Part model, mm, in its own coordinate system. A direction names the side the tool comes from. Round coordinates to 2 decimals unless told otherwise and drop trailing zeros. Write each loop counter-clockwise with the first axis right and the second up, starting at its lowest first coordinate (ties: lowest second). Pieces come first, ordered by that corner, then holes. Notation, with made-up numbers: (81.25, 9) -> (86.25, 9) arc R8 ccw to (86.25, 24) -> close; hole circle Ø10 at (37.5, -2). An arc over 180 degrees is marked (long way). Return JSON: item names as keys, results as strings. Group by question number.
(1) Saw through at D-D (x = -34). List the corners of the cut face in (y, z) (3 decimals), plus the area to 3 significant figures.
(2) Tool access for faces 5 (the cylindrical face through (53.513, -11.795, -23.021)), 6 (the cylindrical face through (-39.05, 11.79, -10.66)), 7 (the flat face through (-53, 0, -22.066)): list every direction of +Z, -Z, +X, -X, +Y, -Y with a clear straight run to the whole face (end or side of a thin tool).
(3) Saw through at A-A (y = 0). State how many separate pieces and enclosed holes the cut face has, plus the area to 3 significant figures.
(4) Drill centre lines: L1, parallel to X at y = 5, z = -6.5; L2, parallel to Y at x = -57, z = -29; L3, parallel to X at y = -2.25, z = -24.5. Where is each one in solid material? Low to high. Write a range as from..to.
(5) Saw through at C-C (z = -6). List the corners of the cut face in (x, y) (3 decimals), plus the area to 3 significant figures.
(6) Drop flat-ended pins along their axis: pin 1 Ø6 at (y, z) = (9.5, 7.5) entering from +X; pin 2 Ø5.5 at (y, z) = (-1, -2) entering from -X; pin 3 Ø7.5 at (x, y) = (-55, 0.5) entering from +Z. Give the stop position or say it passes through.
(7) Mould opens along X. For faces 1 (the flat face through (0, -12.7, 10)), 2 (the cylindrical face through (-39.05, -11.79, -10.66)), 3 (the cylindrical face through (61.59, -10.89, -28.37)), 4 (the cylindrical face through (-49.85, 11.79, -6.46)) say: +X half, -X half, draft (parallel to the pull), parting line (faces both ways), or undercut.
(8) Saw through at B-B (x = 0). List the corners of the cut face in (y, z) (3 decimals).
from build123d import *

# Parameters (mm, degrees)
F1_DEPTH = 12.7
F2_R     = 3.175
F3_DEPTH = 9.526
F4_R     = 6.35
F5_DEPTH = 50.801
F6_R     = 6.35
F7_R     = 3.17499


# Not quite as in the source:
# - a fillet or chamfer is up to 0.001 mm smaller than in the source, because OpenCascade refuses the exact size


with BuildPart() as f1:
    # F0 (on Front) → F1 (new body, symmetric)
    with BuildSketch(Plane.XZ):
        Polygon((-50.8, -22.066242151), (-63.5, -22.066242151), (-63.5, -31.591242151), (-38.1, -31.591242151), (-38.1, 6.508757849), (0, 6.508757849), (38.1, 6.508757849), (38.1, -31.591242151), (63.5, -31.591242151), (63.5, -22.066242151), (50.8, -22.066242151), (50.8, 19.208757849), (0, 19.208757849), (-50.8, 19.208757849), align=None)
    extrude(amount=F1_DEPTH, both=True)

    # F2 (on face) → F3 (cut, through all)
    with BuildSketch(Plane.XY.offset(-22.066242151)):
        with Locations((-57.15, 0)):
            Circle(F2_R)
        with Locations((57.15, 0)):
            Circle(F2_R)
    extrude(amount=-F3_DEPTH, mode=Mode.SUBTRACT)

    # F4 (on face) → F5 (cut, through all)
    with BuildSketch(Plane.XY.offset(19.208757849)):
        Circle(F4_R)
    extrude(amount=-F5_DEPTH, mode=Mode.SUBTRACT)

    # F6
    f6_edges = [f1.edges().sort_by_distance(p)[0] for p in [
        (-50.8, 0, 19.208758),
        (50.8, 0, 19.208758),
        (-63.5, -12.7, -26.828742),
        (63.5, -12.7, -26.828742),
        (63.5, 12.7, -26.828742),
        (-63.5, 12.7, -26.828742),
    ]]
    fillet(f6_edges, radius=F6_R)

    # F7 (radius 3.175 in the source; OpenCascade refuses exactly that, so slightly less here)
    f7_edges = [f1.edges().sort_by_distance(p)[0] for p in [
        (-50.8, -12.7, -4.603742),
        (-53.975, -12.7, -22.066242),
        (-38.1, -12.7, -12.541242),
        (0, -12.7, 6.508758),
        (38.1, -12.7, -12.541242),
        (50.8, 12.7, -4.603742),
        (53.975, 12.7, -22.066242),
        (38.1, 12.7, -12.541242),
        (0, 12.7, 6.508758),
        (-38.1, 12.7, -12.541242),
    ]]
    fillet(f7_edges, radius=F7_R)


solid = f1.part
Computed values:
{
 "1": {"outline": "(-12.7, 9.684) arc R3.175 ccw to (-9.525, 6.509) -> (9.525, 6.509) arc R3.175 ccw to (12.7, 9.684) -> (12.7, 16.034) arc R3.175 ccw to (9.525, 19.209) -> (-9.525, 19.209) arc R3.175 ccw to (-12.7, 16.034) -> close", "area": "314 mm2"},
 "2": {"face 5": "+Z, +X, -Y", "face 6": "-Z, +Y", "face 7": "+Z, -X, +Y, -Y"},
 "3": {"separate pieces": "4", "enclosed holes": "0", "area": "2,200 mm2"},
 "4": {"L1": "-50.8..-38.1, 38.1..50.8", "L2": "-12.7..-3.17, 3.17..12.7", "L3": "-63.41..-59.39, -54.91..-38.1, 38.1..54.91, 59.39..63.41"},
 "5": {"outline": "(-50.8, -9.525) arc R3.175 ccw to (-47.625, -12.7) -> (-41.275, -12.7) arc R3.175 ccw to (-38.1, -9.525) -> (-38.1, 9.525) arc R3.175 ccw to (-41.275, 12.7) -> (-47.625, 12.7) arc R3.175 ccw to (-50.8, 9.525) -> close; (38.1, -9.525) arc R3.175 ccw to (41.275, -12.7) -> (47.625, -12.7) arc R3.175 ccw to (50.8, -9.525) -> (50.8, 9.525) arc R3.175 ccw to (47.625, 12.7) -> (41.275, 12.7) arc R3.175 ccw to (38.1, 9.525) -> close", "area": "628 mm2"},
 "6": {"pin 1": "x = 50.8", "pin 2": "x = -50.8", "pin 3": "z = -22.07"},
 "7": {"face 1": "draft", "face 2": "undercut", "face 3": "+X half", "face 4": "-X half"},
 "8": {"outline": "(-12.7, 9.684) arc R3.175 ccw to (-9.525, 6.509) -> (-6.35, 6.509) -> (-6.35, 19.209) -> (-9.525, 19.209) arc R3.175 ccw to (-12.7, 16.034) -> close; (6.35, 6.509) -> (9.525, 6.509) arc R3.175 ccw to (12.7, 9.684) -> (12.7, 16.034) arc R3.175 ccw to (9.525, 19.209) -> (6.35, 19.209) -> close"}
}
